Autodesk Inventor part; units mm, degrees
ref_plane "YZ Plane" through (0, 0, 0) normal (1, 0, 0) x (0, 1, 0)
ref_plane "XZ Plane" through (0, 0, 0) normal (0, 1, 0) x (-1, 0, 0)
ref_plane "XY Plane" through (0, 0, 0) normal (0, 0, 1) x (1, 0, 0)
sketch "Sketch1" plane through (0, 0, 0) normal (0, 0, 1) x (1, 0, 0)
  line L0 (0, 0) -> (107, 0)
  line L1 (107, 0) -> (107, 36)
  line L2 (107, 36) -> (0, 36)
  line L3 (0, 36) -> (0, 0)
  line L4 (0, 15.75) -> (0, 20.25)
  line L5 (15, 36) -> (35, 36)
  line L6 (35, 36) -> (35, 39)
  line L7 (35, 39) -> (15, 39)
  line L8 (15, 39) -> (15, 36)
  line L9 (65, 36) -> (85, 36)
  line L10 (85, 36) -> (85, 39)
  line L11 (85, 39) -> (65, 39)
  line L12 (65, 39) -> (65, 36)
  line L13 (15, 0) -> (35, 0)
  line L14 (35, 0) -> (35, -3)
  line L15 (35, -3) -> (15, -3)
  line L16 (15, -3) -> (15, 0)
  line L17 (65, 0) -> (85, 0)
  line L18 (85, 0) -> (85, -3)
  line L19 (85, -3) -> (65, -3)
  line L20 (65, -3) -> (65, 0)
  line L21 (5, 20.25) -> (13, 20.25)
  line L22 (13, 20.25) -> (13, 15.75)
  line L23 (13, 15.75) -> (5, 15.75)
  line L24 (5, 15.75) -> (5, 20.25)
  line L25 (94, 20.25) -> (102, 20.25)
  line L26 (102, 20.25) -> (102, 15.75)
  line L27 (102, 15.75) -> (94, 15.75)
  line L28 (94, 15.75) -> (94, 20.25)
  point P0 (102, 18)
  dimension "d0" = 36
  dimension "d1" = 107
  dimension "d6" = 3
  dimension "d7" = 3
  dimension "d8" = 30
  dimension "d9" = 20
  dimension "d10" = 20
  dimension "d11" = 15
  dimension "d14" = 4.5
  dimension "d15" = 8
  dimension "d16" = 8
  dimension "d18" = 97
  dimension "d19" = 5
  dimension "d20" = 18
extrude "Extrusion1" add sketch "Sketch1" along normal blind 3
properties part number "TB6600holder"
Build history of the part. All positions in model axes, mm. A direction names the side the tool comes from. Round coordinates to 2 decimals unless told otherwise and drop trailing zeros. Write each loop counter-clockwise with the first axis right and the second up, starting at its lowest first coordinate (ties: lowest second). Pieces come first, ordered by that corner, then holes.
1) Drill centre lines: probe 1 along X at (y, z) = (19, 1.2); probe 2 along X at (y, z) = (37, 1.05); probe 3 along Y at (x, z) = (101, 0.75). Where is each one in solid material? Low to high.
2) Mould opens along X. For faces 5 (the flat face through (0, 18, 1)), 6 (the flat face through (13, 18, 1)), 7 (the flat face through (65, -2, 1)), 8 (the flat face through (53, 18, 3)) say: +X half, -X half, draft (parallel to the pull), parting line (faces both ways), or undercut.
3) Band-saw the part on C-C, the plane x = 55.5. List the corners of the cut face in (y, z), and give its area (3 significant figures).
4) Band-saw the part on A-A, the plane x = 9. List the corners of the cut face in (y, z).
5) 3-axis set-ups, long thin cutter, end or side, ignore diameter. For faces 1 (the flat face through (96, 0, 1)), 2 (the flat face through (9, 20.25, 1)), 3 (the flat face through (35, 37, 1)), 4 (the flat face through (8, 36, 1)): which of +Z, -Z, +X, -X, +Y, -Y reach the whole face in a straight line?
6) Band-saw the part on B-B, the plane z = 1.35. List the corners of the cut face in (x, y), and give its area (3 significant figures).
7) Pin check, flat tips, straight feed: pin 1 (1.5 mm diameter, centred on y = -1, z = 1, fed in from -X); pin 2 (4 mm diameter, centred on x = 95, y = 17.5, fed in from +Z); pin 3 (1.5 mm diameter, centred on y = -1.5, z = 2, fed in from +X); pin 4 (1.5 mm diameter, centred on x = 7, z = 1.5, fed in from -Y). Stop position of each tip, or through.
Ans:
1. probe 1: x = 0 to 5, 13 to 94, 102 to 107
1. probe 2: x = 15 to 35, 65 to 85
1. probe 3: y = 0 to 15.75, 20.25 to 36
2. face 5: -X half
2. face 6: undercut
2. face 7: undercut
2. face 8: draft
3. outline: (0, 0) - (36, 0) - (36, 3) - (0, 3) - close
3. area: 108 mm2
4. outline: (0, 0) - (15.75, 0) - (15.75, 3) - (0, 3) - close; (20.25, 0) - (36, 0) - (36, 3) - (20.25, 3) - close
5. face 1: +Z, -Z, +X, -Y
5. face 2: +Z, -Z
5. face 3: +Z, -Z, +Y
5. face 4: +Z, -Z, -X, +Y
6. outline: (0, 0) - (15, 0) - (15, -3) - (35, -3) - (35, 0) - (65, 0) - (65, -3) - (85, -3) - (85, 0) - (107, 0) - (107, 36) - (85, 36) - (85, 39) - (65, 39) - (65, 36) - (35, 36) - (35, 39) - (15, 39) - (15, 36) - (0, 36) - close; hole (5, 15.75) - (13, 15.75) - (13, 20.25) - (5, 20.25) - close; hole (94, 15.75) - (102, 15.75) - (102, 20.25) - (94, 20.25) - close
6. area: 4,020 mm2
7. pin 1: stops at x = 15
7. pin 2: stops at z = 3
7. pin 3: stops at x = 85
7. pin 4: stops at y = 0
